CAD build for the part. Positions are in the model's coordinates, mm. A direction names the side the tool comes from. Coordinates: 2 decimals unless noted, no trailing zeros. Write each loop counter-clockwise with the first axis right and the second up, starting at its lowest first coordinate (ties: lowest second). Pieces come first, ordered by that corner, then holes. Notation, with made-up numbers: M -20,-17 L 9,-17 A21 cw 9,-10 Z; hole C 75.25,-25.75 d4. An arc over 180 degrees is marked long. Answer as CSV lines item,"result". Start each with the question number.
```python
from build123d import *

# Parameters (mm, degrees)
SKETCH001_W     = 299
SKETCH001_H     = 109
PAD_DEPTH       = 6
SKETCH002_W     = 287
SKETCH002_H     = 97
POCKET_DEPTH    = 4
SKETCH003_W     = 299
SKETCH003_H     = 109
SKETCH003_W_2   = 294.96
SKETCH003_H_2   = 104.96
POCKET001_DEPTH = 3
SKETCH004_W     = 80
SKETCH004_H     = 4
SKETCH004_W_2   = 4
SKETCH004_H_2   = 32.5
POCKET002_DEPTH = 1.25
SKETCH_W        = 13
SKETCH_H        = 6
POCKET003_DEPTH = 4
FILLET_R        = 0.99
FILLET001_R     = 0.99


with BuildPart() as part:
    # Sketch001 → Pad (new body)
    with BuildSketch(Plane.XY):
        Rectangle(SKETCH001_W, SKETCH001_H)
    extrude(amount=PAD_DEPTH)

    # Sketch002 (on Face6 of Pad) → Pocket (cut)
    with BuildSketch(Plane.XY.offset(6)):
        Rectangle(SKETCH002_W, SKETCH002_H)
    extrude(amount=-POCKET_DEPTH, mode=Mode.SUBTRACT)

    # Sketch003 (on Face5 of Pocket) → Pocket001 (cut)
    with BuildSketch(Plane.XY.offset(6)):
        Rectangle(SKETCH003_W, SKETCH003_H)
        Rectangle(SKETCH003_W_2, SKETCH003_H_2, mode=Mode.SUBTRACT)
    extrude(amount=-POCKET001_DEPTH, mode=Mode.SUBTRACT)

    # Sketch004 (on Face11 of Pocket001) → Pocket002 (cut)
    with BuildSketch(Plane.XY.offset(6)):
        with Locations((-94.580218, 50.5)):
            Rectangle(SKETCH004_W, SKETCH004_H)
        with Locations((0.419782, 50.5)):
            Rectangle(SKETCH004_W, SKETCH004_H)
        with Locations((95.419782, 50.5)):
            Rectangle(SKETCH004_W, SKETCH004_H)
        with Locations((96.548097, -50.5)):
            Rectangle(SKETCH004_W, SKETCH004_H)
        with Locations((1.548097, -50.5)):
            Rectangle(SKETCH004_W, SKETCH004_H)
        with Locations((-93.451903, -50.5)):
            Rectangle(SKETCH004_W, SKETCH004_H)
        with Locations((-145.5, 23.75)):
            Rectangle(SKETCH004_W_2, SKETCH004_H_2)
        with Locations((-145.5, -23.75)):
            Rectangle(SKETCH004_W_2, SKETCH004_H_2)
        with Locations((145.5, 23.75)):
            Rectangle(SKETCH004_W_2, SKETCH004_H_2)
        with Locations((145.5, -23.75)):
            Rectangle(SKETCH004_W_2, SKETCH004_H_2)
    extrude(amount=-POCKET002_DEPTH, mode=Mode.SUBTRACT)

    # Sketch (on Face43 of Pocket002) → Pocket003 (cut)
    with BuildSketch(Plane.XY.offset(6)):
        with Locations((-124, 51.5)):
            Rectangle(SKETCH_W, SKETCH_H)
    extrude(amount=-POCKET003_DEPTH, mode=Mode.SUBTRACT)

    # Fillet
    fillet_edges = [part.edges().sort_by_distance(p)[0] for p in [
        (-130.5, 51.5, 2),
    ]]
    fillet(fillet_edges, radius=FILLET_R)

    # Fillet001
    fillet001_edges = [part.edges().sort_by_distance(p)[0] for p in [
        (-117.5, 51.5, 2),
    ]]
    fillet(fillet001_edges, radius=FILLET001_R)


solid = part.part
```
1) Band-saw the part on A-A, the plane x = 127. List the corners of the cut face in (y, z), plus the area to 3 significant figures.
2) Band-saw the part on B-B, the plane y = -26. List the corners of the cut face in (x, z).
3) Pin check, flat tips, straight feed: P1, Ø0.9, axis at x = -6, z = 5, coming from the -Y side; P2, Ø1, axis at x = -146, z = 5.5, coming from the +Y side; P3, Ø0.6, axis at y = -50, z = 5.5, coming from the -X side. Stop position of each tip, or through.
4) Probe L1, parallel to Y at x = -89, z = 3.75; L2, parallel to Y at x = 48, z = 2.65; L3, parallel to Z at x = -58, y = 47.5. List the from-to ranges inside material, lowest first. Write a range as [from, to].
5) Tool access for faces 1 (the flat face through (144, 48, 6)), 2 (the flat face through (-2, -8, 2)): list every direction of +Z, -Z, +X, -X, +Y, -Y with a clear straight run to the whole face (end or side of a thin tool).
Result sheet:
1,outline,"M -54.5,0 L 54.5,0 L 54.5,3 L 52.48,3 L 52.48,4.75 L 48.5,4.75 L 48.5,2 L -48.5,2 L -48.5,4.75 L -52.48,4.75 L -52.48,3 L -54.5,3 Z"
1,area,"244 mm²"
2,outline,"M -149.5,0 L 149.5,0 L 149.5,3 L 147.48,3 L 147.48,4.75 L 143.5,4.75 L 143.5,2 L -143.5,2 L -143.5,4.75 L -147.48,4.75 L -147.48,3 L -149.5,3 Z"
3,P1,"stops at y = -52.48"
3,P2,"stops at y = 52.48"
3,P3,"stops at x = -147.48"
4,L1,"y = [-52.48, -48.5], [48.5, 52.48]"
4,L2,"y = [-54.5, -48.5], [48.5, 54.5]"
4,L3,"z = [0, 2]"
5,face 1,"+Z, +X, -X, +Y, -Y"
5,face 2,"+Z"
